```python
from build123d import *

# Parameters (mm, degrees)
SKETCH1_W           = 30
SKETCH1_H           = 28
SKETCH1_R           = 11
BOSS_EXTRUDE1_DEPTH = 7
SKETCH2_W           = 5
SKETCH2_H           = 2.5
BOSS_EXTRUDE2_DEPTH = 13
CHAMFER2_SIZE       = 2
BOSS_EXTRUDE6_DEPTH = 2.5
CHAMFER3_SIZE       = 2
CHAMFER4_SIZE       = 2
BOSS_EXTRUDE4_DEPTH = 2.5
CHAMFER6_SIZE       = 2.5
CHAMFER7_SIZE       = 7
CHAMFER7_SIZE_2     = 13.165085257
SKETCH7_R           = 1.5
CUT_EXTRUDE2_DEPTH  = 6.4
BOSS_EXTRUDE7_START = -2.5
SKETCH8_W           = 30
SKETCH8_H           = 5
BOSS_EXTRUDE7_DEPTH = 4.5
CHAMFER8_SIZE       = 4.000836323
CHAMFER8_SIZE_2     = 2.5


with BuildPart() as part:
    # Sketch1 → Boss-Extrude1 (new body)
    with BuildSketch(Plane.XY):
        Rectangle(SKETCH1_W, SKETCH1_H)
        Circle(SKETCH1_R, mode=Mode.SUBTRACT)
    extrude(amount=BOSS_EXTRUDE1_DEPTH)

    # Sketch2 → Boss-Extrude2 (add)
    with BuildSketch(Plane(origin=(0, 0, 0), x_dir=(-1, 0, 0), z_dir=(0, 0, -1))):
        with Locations((-12.5, -12.75)):
            Rectangle(SKETCH2_W, SKETCH2_H)
        with Locations((12.5, -12.75)):
            Rectangle(SKETCH2_W, SKETCH2_H)
    extrude(amount=BOSS_EXTRUDE2_DEPTH)

    # Chamfer2
    chamfer2_edges = [part.edges().sort_by_distance(p)[0] for p in [
        (-10, -12.75, 0),
        (10, -12.75, 0),
    ]]
    chamfer(chamfer2_edges, length=CHAMFER2_SIZE)

    # Sketch5 → Boss-Extrude6 (add)
    with BuildSketch(Plane.XZ.offset(14)):
        Polygon((-10, -2), (-10, -7.5), (10, -7.5), (10, -2), (8, 0), (-8, 0), align=None)
    extrude(amount=-BOSS_EXTRUDE6_DEPTH)

    # Chamfer3
    chamfer3_edges = [part.edges().sort_by_distance(p)[0] for p in [
        (15, 0, 7),
    ]]
    chamfer(chamfer3_edges, length=CHAMFER3_SIZE)

    # Chamfer4
    chamfer4_edges = [part.edges().sort_by_distance(p)[0] for p in [
        (-15, 0, 7),
    ]]
    chamfer(chamfer4_edges, length=CHAMFER4_SIZE)

    # Sketch4 → Boss-Extrude4 (add)
    with BuildSketch(Plane(origin=(0, 0, 0), x_dir=(-1, 0, 0), z_dir=(0, 0, -1))):
        Polygon((-15, 0), (15, 11.5), (15, 14), (-15, 14), align=None)
    extrude(amount=BOSS_EXTRUDE4_DEPTH)

    # Chamfer6
    # the kernel refuses this chamfer: 2.5 mm, written as the material it adds along each edge
    with BuildSketch(Plane(origin=(21.003247512, -2.30124488, 0), x_dir=(-0.3578006820796162, -0.9333930836859554, 0.02749587661058638), z_dir=(-0.9337461173020497, 0.35793601163245237, 0))) as chamfer6_piece_1_section:
        Polygon((CHAMFER6_SIZE * 0.999621916911, -CHAMFER6_SIZE * 0.0274958766106), (-CHAMFER6_SIZE * 0.0274958766106, -CHAMFER6_SIZE * 0.999621916911), (0, 0), align=None)
    chamfer6_piece_1 = extrude(amount=17.263908412, mode=Mode.PRIVATE)
    chamfer6_piece_1 = chamfer6_piece_1 - Plane(origin=(0, 0, -0.835393566), x_dir=(1, 0, 0), z_dir=(0, 0, -1)) * Cylinder(11, 45, mode=Mode.PRIVATE)
    chamfer6_piece_1 = split(chamfer6_piece_1, bisect_by=Plane(origin=(15, -0.113968884, -0.835393566), z_dir=(-1, 0, 0)), keep=Keep.TOP, mode=Mode.PRIVATE)
    add(chamfer6_piece_1)
    with BuildSketch(Plane(origin=(-1.03959441, 6.148511191, 0), x_dir=(-0.35780068207961624, -0.9333930836859554, 0.02749587661058638), z_dir=(-0.9337461173020497, 0.35793601163245237, 0))) as chamfer6_piece_2_section:
        Polygon((CHAMFER6_SIZE * 0.999621916911, -CHAMFER6_SIZE * 0.0274958766106), (-CHAMFER6_SIZE * 0.0274958766106, -CHAMFER6_SIZE * 0.999621916911), (0, 0), align=None)
    chamfer6_piece_2 = extrude(amount=21.380172546, mode=Mode.PRIVATE)
    chamfer6_piece_2 = chamfer6_piece_2 - Plane(origin=(0, 0, -0.851534645), x_dir=(1, 0, 0), z_dir=(0, 0, -1)) * Cylinder(11, 53, mode=Mode.PRIVATE)
    chamfer6_piece_2 = split(chamfer6_piece_2, bisect_by=Plane(origin=(-15, 9.244820467, -0.851534645), z_dir=(1, 0, 0)), keep=Keep.TOP, mode=Mode.PRIVATE)
    add(chamfer6_piece_2)

    # Chamfer7
    # the kernel refuses this chamfer: 13.165085257, 7 mm, written as the material it adds along each edge
    with BuildSketch(Plane(origin=(-15, -11.5, 0), x_dir=(0, 0.9979482451756082, 0.06402577567608186), z_dir=(1, 0, 0))) as chamfer7_piece_1_section:
        Polygon((CHAMFER7_SIZE * 0.997948245176, -CHAMFER7_SIZE * 0.0640257756761), (-CHAMFER7_SIZE_2 * 0.0640257756781, -CHAMFER7_SIZE_2 * 0.997948245208), (0, 0), align=None)
    chamfer7_piece_1 = extrude(amount=30, mode=Mode.PRIVATE)
    chamfer7_piece_1 = chamfer7_piece_1 - Plane(origin=(0, 0, -3.073682767), x_dir=(1, 0, 0), z_dir=(0, 0, -1)) * Cylinder(11, 113, mode=Mode.PRIVATE)
    chamfer7_piece_1 = split(chamfer7_piece_1, bisect_by=Plane(origin=(-10, -8.887755394, -3.073682767), z_dir=(-1, 0, 0)), keep=Keep.TOP, mode=Mode.PRIVATE)
    chamfer7_piece_1 = split(chamfer7_piece_1, bisect_by=Plane(origin=(-12.500128058, -8.887755394, -7.5), z_dir=(0, 0, 1)), keep=Keep.TOP, mode=Mode.PRIVATE)
    add(chamfer7_piece_1)
    with BuildSketch(Plane(origin=(-15, -11.5, 0), x_dir=(0, 0.9979482451756082, 0.06402577567608186), z_dir=(1, 0, 0))) as chamfer7_piece_2_section:
        Polygon((CHAMFER7_SIZE * 0.997948245176, -CHAMFER7_SIZE * 0.0640257756761), (-CHAMFER7_SIZE_2 * 0.0640257756781, -CHAMFER7_SIZE_2 * 0.997948245208), (0, 0), align=None)
    chamfer7_piece_2 = extrude(amount=30, mode=Mode.PRIVATE)
    chamfer7_piece_2 = split(chamfer7_piece_2, bisect_by=Plane(origin=(-10, -10.721530873, -9.597564575), z_dir=(-1, 0, 0)), keep=Keep.TOP, mode=Mode.PRIVATE)
    chamfer7_piece_2 = split(chamfer7_piece_2, bisect_by=Plane(origin=(-12.5, -10.721530873, -7.5), z_dir=(0, 0, -1)), keep=Keep.TOP, mode=Mode.PRIVATE)
    chamfer7_piece_2 = split(chamfer7_piece_2, bisect_by=Plane(origin=(-12.5, -10.721530873, -13), z_dir=(0, 0, 1)), keep=Keep.TOP, mode=Mode.PRIVATE)
    add(chamfer7_piece_2)
    with BuildSketch(Plane(origin=(-15, -11.5, 0), x_dir=(0, 0.9979482451756082, 0.06402577567608186), z_dir=(1, 0, 0))) as chamfer7_piece_3_section:
        Polygon((CHAMFER7_SIZE * 0.997948245176, -CHAMFER7_SIZE * 0.0640257756761), (-CHAMFER7_SIZE_2 * 0.0640257756781, -CHAMFER7_SIZE_2 * 0.997948245208), (0, 0), align=None)
    chamfer7_piece_3 = extrude(amount=30, mode=Mode.PRIVATE)
    chamfer7_piece_3 = chamfer7_piece_3 - Plane(origin=(0, 0, -3.793876077), x_dir=(1, 0, 0), z_dir=(0, 0, -1)) * Cylinder(11, 113, mode=Mode.PRIVATE)
    chamfer7_piece_3 = split(chamfer7_piece_3, bisect_by=Plane(origin=(-10, -6.598719884, -3.793876077), z_dir=(1, 0, 0)), keep=Keep.TOP, mode=Mode.PRIVATE)
    chamfer7_piece_3 = split(chamfer7_piece_3, bisect_by=Plane(origin=(-9.499486782, -6.598719884, -7.5), z_dir=(0, 0, 1)), keep=Keep.TOP, mode=Mode.PRIVATE)
    chamfer7_piece_3 = split(chamfer7_piece_3, bisect_by=Plane(origin=(10, -6.598719884, -3.793876077), z_dir=(-1, 0, 0)), keep=Keep.TOP, mode=Mode.PRIVATE)
    add(chamfer7_piece_3)
    with BuildSketch(Plane(origin=(-15, -11.5, 0), x_dir=(0, 0.9979482451756082, 0.06402577567608186), z_dir=(1, 0, 0))) as chamfer7_piece_4_section:
        Polygon((CHAMFER7_SIZE * 0.997948245176, -CHAMFER7_SIZE * 0.0640257756761), (-CHAMFER7_SIZE_2 * 0.0640257756781, -CHAMFER7_SIZE_2 * 0.997948245208), (0, 0), align=None)
    chamfer7_piece_4 = extrude(amount=30, mode=Mode.PRIVATE)
    chamfer7_piece_4 = split(chamfer7_piece_4, bisect_by=Plane(origin=(12.5, -10.721530873, -7.5), z_dir=(0, 0, -1)), keep=Keep.TOP, mode=Mode.PRIVATE)
    chamfer7_piece_4 = split(chamfer7_piece_4, bisect_by=Plane(origin=(10, -10.721530873, -9.597564575), z_dir=(1, 0, 0)), keep=Keep.TOP, mode=Mode.PRIVATE)
    chamfer7_piece_4 = split(chamfer7_piece_4, bisect_by=Plane(origin=(12.5, -10.721530873, -13), z_dir=(0, 0, 1)), keep=Keep.TOP, mode=Mode.PRIVATE)
    add(chamfer7_piece_4)
    with BuildSketch(Plane(origin=(-15, -11.5, 0), x_dir=(0, 0.9979482451756082, 0.06402577567608186), z_dir=(1, 0, 0))) as chamfer7_piece_5_section:
        Polygon((CHAMFER7_SIZE * 0.997948245176, -CHAMFER7_SIZE * 0.0640257756761), (-CHAMFER7_SIZE_2 * 0.0640257756781, -CHAMFER7_SIZE_2 * 0.997948245208), (0, 0), align=None)
    chamfer7_piece_5 = extrude(amount=30, mode=Mode.PRIVATE)
    chamfer7_piece_5 = chamfer7_piece_5 - Plane(origin=(0, 0, -3.073682766), x_dir=(1, 0, 0), z_dir=(0, 0, -1)) * Cylinder(11, 113, mode=Mode.PRIVATE)
    chamfer7_piece_5 = split(chamfer7_piece_5, bisect_by=Plane(origin=(12.500128057, -8.887755394, -7.5), z_dir=(0, 0, 1)), keep=Keep.TOP, mode=Mode.PRIVATE)
    chamfer7_piece_5 = split(chamfer7_piece_5, bisect_by=Plane(origin=(10, -8.887755394, -3.073682766), z_dir=(1, 0, 0)), keep=Keep.TOP, mode=Mode.PRIVATE)
    add(chamfer7_piece_5)

    # Sketch7 → Cut-Extrude2 (cut)
    with BuildSketch(Plane.XZ.offset(14)):
        with Locations(Location((-11, 2.5, 0), (0, 0, 270))):
            Circle(SKETCH7_R)
        with Locations(Location((11, 2.5, 0), (0, 0, 270))):
            Circle(SKETCH7_R)
    extrude(amount=-CUT_EXTRUDE2_DEPTH, mode=Mode.SUBTRACT)

    # Sketch8 → Boss-Extrude7 (add)
    with BuildSketch(Plane(origin=(0, 14, 0), x_dir=(1, 0, 0), z_dir=(0, 1, 0)).offset(BOSS_EXTRUDE7_START)):
        with Locations((0, 5)):
            Rectangle(SKETCH8_W, SKETCH8_H)
    extrude(amount=BOSS_EXTRUDE7_DEPTH)

    # Chamfer8
    # the kernel refuses this chamfer: 4.000836323, 2.5 mm, written as the material it adds along each edge
    with BuildSketch(Plane(origin=(-25.343554005, 11.5, -2.5), x_dir=(0, -0.9997899140358645, 0.02049701910421793), z_dir=(1, 0, 0))) as chamfer8_piece_1_section:
        Polygon((CHAMFER8_SIZE * 0.999789913937, CHAMFER8_SIZE * 0.0204970191022), (-CHAMFER8_SIZE_2 * 0.0204970191042, CHAMFER8_SIZE_2 * 0.999789914036), (0, 0), align=None)
    chamfer8_piece_1 = extrude(amount=40.343554005, mode=Mode.PRIVATE)
    chamfer8_piece_1 = split(chamfer8_piece_1, bisect_by=Plane(origin=(2.975759377, 8.202968449, -5.855581208), z_dir=(0.25309898105600476, 0.6602582114512465, 0.707106781186274)), keep=Keep.TOP, mode=Mode.PRIVATE)
    add(chamfer8_piece_1)


solid = part.part
```
Could you check a few things on this model? Use its own coordinates, in mm. A direction names the side the tool comes from. Coordinates: 2 decimals unless noted, no trailing zeros. Write each loop counter-clockwise with the first axis right and the second up, starting at its lowest first coordinate (ties: lowest second). Pieces come first, ordered by that corner, then holes. Notation, with made-up numbers: (-16.5, -24.5) -> (17.5, -24.5) arc R19 cw to (17.5, -7.5) -> close; hole circle Ø5 at (62, 44). An arc over 180 degrees is marked (long way). Write item = value, one per line. Start each with the question number.
(1) Which directions (+Z, -Z, +X, -X, +Y, -Y) give clear straight access to the entire face, cutting with the end or side of a thin tool? Please do faces 1 (the face through (-1.733, -10.863, 1.26)), 2 (the face through (8, 5, -2.5)), 3 (the face through (10, -12, -10)), 4 (the face through (-13, 2, 0)), 5 (the face through (-12.33, -10.84, 1.81)).
(2) I need wall thicknesses on line 1 (X direction, y = -12, z = 2.5); line 2 (X direction, y = -0.25, z = 2); line 3 (Z direction, x = 7, y = 6). Which ranges of each line are inside material? Lowest first, please. Write a range as [from, to].
(3) I want a section at C-C (y = 4). Please give me the cut outline in (x, z), plus the area to 3 significant figures.
(4) I want a section at A-A (x = 0). Please give me the cut outline in (y, z), plus the area to 3 significant figures.
(5) Will these pins go through, and if not, where does the flat tip stop? pin 1 (3 mm diameter, centred on x = -2, y = -11, fed in from -Z); pin 2 (2.5 mm diameter, centred on x = 10.5, z = 3, fed in from -Y); pin 3 (5 mm diameter, centred on x = 11, z = 2.5, fed in from +Y); pin 4 (4 mm diameter, centred on x = -0.5, y = 2.5, fed in from +Z).
(6) I want a section at D-D (y = -10.25). Please give me the cut outline in (x, z).
(7) I want a section at B-B (z = 2.5). Please give me the cut outline in (x, y).
(8) We'd pull the mould along Y, two halves only. Please class faces 6 (the face through (0, 16, -5)), 7 (the face through (0, 14, -7.5)), 8 (the face through (11.83, -7.91, -6.41)): released by +Y, released by -Y, zero draft, split by the parting line, or undercut.
Result set:
q1.face_1 = +Z
q1.face_2 = -Z, +X, -X
q1.face_3 = -Z, +Y, -Y
q1.face_4 = -Z, -X
q1.face_5 = -Y
q2.line_1 = [-15, -12.5], [-9.5, 9.5], [12.5, 15]
q2.line_2 = [-15, -11], [11, 15]
q2.line_3 = [-2.5, 0]
q3.outline = (-15, 0) -> (-10.25, 0) -> (-10.25, 7) -> (-13, 7) -> (-15, 5) -> close; (4.57, -2.5) -> (15, -2.5) -> (15, 5) -> (13, 7) -> (10.25, 7) -> (10.25, 0) -> (4.57, 0) -> close
q3.area = 88.6 mm2
q4.outline = (-14, -7.5) -> (-11, -7.5) -> (-11, 7) -> (-14, 7) -> close; (5.75, -2.5) -> (7.5, -2.5) -> (11.5, -5) -> (11.5, -7.5) -> (16, -7.5) -> (16, -2.5) -> (14, -2.5) -> (14, 7) -> (11, 7) -> (11, 0) -> (5.75, 0) -> close
q4.area = 113 mm2
q5.pin_1 = -7.5
q5.pin_2 = -14
q5.pin_3 = 14
q5.pin_4 = through
q6.outline = (-15, -10.81) -> (-10, -10.81) -> (-10, -7.5) -> (-3.99, -7.5) -> (-3.99, 7) -> (-13, 7) -> (-15, 5) -> close; (3.99, -7.5) -> (10, -7.5) -> (10, -10.81) -> (15, -10.81) -> (15, 5) -> (13, 7) -> (3.99, 7) -> close; hole circle Ø3 at (-11, 2.5); hole circle Ø3 at (11, 2.5)
q7.outline = (-15, -14) -> (-12.5, -14) -> (-12.5, -7.6) -> (-9.5, -7.6) -> (-9.5, -14) -> (9.5, -14) -> (9.5, -7.6) -> (12.5, -7.6) -> (12.5, -14) -> (15, -14) -> (15, 14) -> (-15, 14) -> close; hole circle Ø22 at (0, 0)
q8.face_6 = released by +Y
q8.face_7 = zero draft
q8.face_8 = undercut
